Geometry: final body of the model. Coordinates: model frame, mm. Give positions to 0.01 mm unless a question says otherwise; leave off trailing zeros. Order: outer loops, then holes, each group sorted by start corner. A loop starts at its lowest first (then second) coordinate and runs counter-clockwise, first axis right, second up. Notation, with made-up numbers: (-12.75, -18) -> (46.25, -18) arc R28 ccw to (46.25, 19) -> close; hole circle Ø2 at (-9.5, 87). An arc over 180 degrees is marked (long way). Answer in a Markdown table with one row per item. Add a question column.
Q1. Contact query for a flat-ended pin moving along its axis: P1, Ø3, axis at x = -19.41, z = 9.14, coming from the -Y side. Output: stop coordinate, or through.
Q2. Cut plane C-C on x = 21.5. Return the cut outline in (y, z).
Q3. Pull-direction query (X, two-part tool) for faces 1 (the face through (30, -1, 0)), 2 (the face through (-14.43, -1.38, -6.84)), 3 (the face through (0, -2.8, 0)); classes: +X half, -X half, draft (parallel to the pull), parting line (faces both ways), or undercut.
Q4. Line query: line 1 along X through (y, z) = (-2.55, 9); line 2 along X through (y, z) = (-1, -7); line 3 along X through (y, z) = (-0.7, 0). Output: solid intervals per line, ascending. Write a range as from..to.
Q5. Cut plane A-A on y = -2. Count the separate pieces of the cut face and the enclosed holes in it, and give its area (3 significant figures).
Q6. Cut plane B-B on z = 0. Return the cut outline in (x, y), and give its area (3 significant figures).
from build123d import *

# Parameters (mm, degrees)
F0_W          = 60
F0_H          = 26.8
F1_DEPTH      = 2.8
F2_R          = 1.75
F2_R_2        = 6
F3_DEPTH      = 25
F3_DEPTH_BACK = 25


with BuildPart() as f1:
    # F0 (on Front) → F1 (new body)
    with BuildSketch(Plane.XZ):
        Rectangle(F0_W, F0_H)
    extrude(amount=F1_DEPTH)

    # F2 (on Front) → F3 (cut, two sides)
    with BuildSketch(Plane.XZ) as f3_sk:
        with Locations((-19.407583, 9.143958)):
            Circle(F2_R)
        with Locations((-21.087086, 3.172394)):
            Circle(F2_R)
        with Locations((-16.981635, 5.225119)):
            Circle(F2_R)
        with Locations((-16.839717, 0.773296)):
            Circle(F2_R)
        with Locations((-20.605817, -2.600502)):
            Circle(F2_R)
        with Locations((-16.055113, -4.09125)):
            Circle(F2_R)
        with Locations((-13.622839, 8.93318)):
            Circle(F2_R)
        with Locations((-12.681315, 2.813267)):
            Circle(F2_R)
        with Locations((-11.89671, -2.522042)):
            Circle(F2_R)
        with Locations((-12.681315, -6.915826)):
            Circle(F2_R)
        with Locations((-20.841198, -6.915826)):
            Circle(F2_R)
        with Locations((-16.761256, -9.269638)):
            Circle(F2_R)
        with Locations((16.035197, 0)):
            Circle(F2_R_2)
        with Locations((-10.051827, 6.095069)):
            Circle(F2_R)
        with Locations((-24.795463, 0)):
            Circle(F2_R)
        with Locations((-24.105322, 6.147532)):
            Circle(F2_R)
        with Locations((-7.508276, -5.214532)):
            Circle(F2_R)
    extrude(amount=F3_DEPTH, mode=Mode.SUBTRACT)
    extrude(f3_sk.sketch, amount=-F3_DEPTH_BACK, mode=Mode.SUBTRACT)


solid = f1.part
Completed:
| question | item | result |
|---|---|---|
| 1 | P1 | passes through |
| 2 | outline | (-2.8, -13.4) -> (0, -13.4) -> (0, -2.48) -> (-2.8, -2.48) -> close; (-2.8, 2.48) -> (0, 2.48) -> (0, 13.4) -> (-2.8, 13.4) -> close |
| 3 | face 1 | +X half |
| 3 | face 2 | undercut |
| 3 | face 3 | draft |
| 4 | line 1 | x = -30..-21.15, -17.66..-15.37, -11.87..30 |
| 4 | line 2 | x = -30..-22.59, -19.09..-14.43, -10.93..30 |
| 4 | line 3 | x = -30..-26.55, -23.05..-18.41, -15.27..10.04, 22.04..30 |
| 5 | separate pieces | 1 |
| 5 | enclosed holes | 17 |
| 5 | area | 1,340 mm² |
| 6 | outline | (-30, -2.8) -> (-26.55, -2.8) -> (-26.55, 0) -> (-30, 0) -> close; (-23.05, -2.8) -> (-18.41, -2.8) -> (-18.41, 0) -> (-23.05, 0) -> close; (-15.27, -2.8) -> (10.04, -2.8) -> (10.04, 0) -> (-15.27, 0) -> close; (22.04, -2.8) -> (30, -2.8) -> (30, 0) -> (22.04, 0) -> close |
| 6 | area | 116 mm² |
